Study the drawing (mm; zero at the part's minimum x, y, z) and answer. A direction names the side the tool comes from. Coordinates: 2 decimals unless noted, no trailing zeros. Write each loop counter-clockwise with the first axis right and the second up, starting at its lowest first coordinate (ties: lowest second). Pieces come first, ordered by that corner, then holes. Notation, with made-up numbers: (15, 16) -> (36, 16) arc R10 cw to (36, 24) -> close; hole circle Ø10 at (-21, -28). An arc over 180 degrees is marked (long way). Answer in a Markdown table with one row per item. Add a question column.
Item 1: For a pull along Y with two mould halves and no side action, classify the marked faces 1, 2 and 3 as +Y half, -Y half, draft (parallel to the pull), parting line (faces both ways), or undercut.
Item 2: Which of the six approach directions +Z, -Z, +X, -X, +Y, -Y give full straight-line access (tool end or side, diameter ignored) to the marked faces 4 and 5?
Item 3: Section B-B on z = 25 is taken. Write down the section's boundary in (x, y), then the cut area to 3 significant figures.
Item 4: Section D-D on x = 2 is taken. Write down the section's boundary in (y, z).
Item 5: Section C-C on y = 12.5 is taken. Write down the section's boundary in (x, z).
Item 6: Straight lines are drawn through the part: line 1 (Y direction, x = 8, z = 12.25); line 2 (Z direction, x = 5, y = 1); line 3 (Y direction, x = 9.75, z = 22) (1 decimal). For each, find the intervals that lie inside material, in ascending order. Write a range as from..to.
Item 7: Given pin 1 Ø3 at (x, z) = (7.5, 14) entering from -Y; pin 2 Ø1.5 at (x, y) = (7.5, 7) entering from -Z; pin 3 Ø1.5 at (x, z) = (6.5, 16) entering from -Y (1 decimal), each flat-ended and moving along its own axis, determine where each tip first touches the part or whether it passes through.
Item 8: Section A-A on x = 8 is taken. Write down the section's boundary in (y, z).
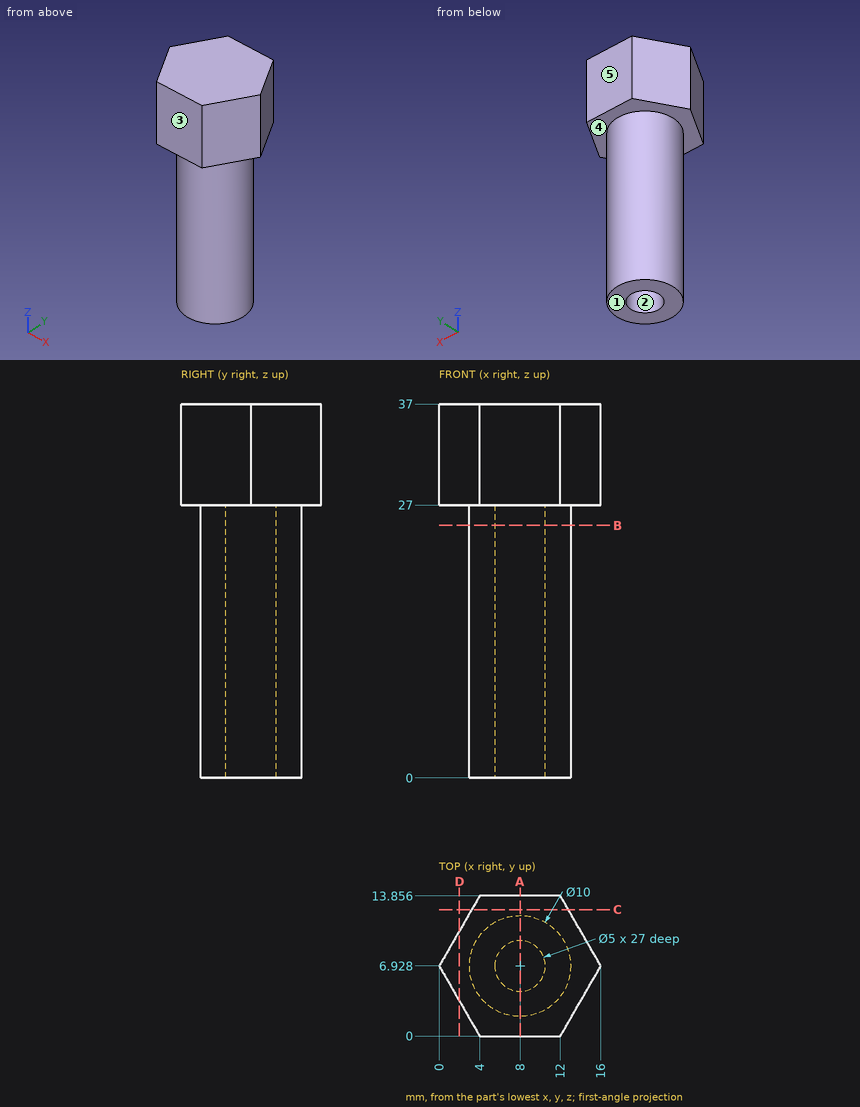
Results below:
| question | item | result |
|---|---|---|
| 1 | face 1 | draft |
| 1 | face 2 | undercut |
| 1 | face 3 | -Y half |
| 2 | face 4 | -Z |
| 2 | face 5 | +Z, -Z, +X, -X, +Y |
| 3 | outline | circle Ø10 at (8, 6.93); hole circle Ø5 at (8, 6.93) |
| 3 | area | 58.9 mm2 |
| 4 | outline | (3.46, 27) -> (10.39, 27) -> (10.39, 37) -> (3.46, 37) -> close |
| 5 | outline | (3.22, 27) -> (12.78, 27) -> (12.78, 37) -> (3.22, 37) -> close |
| 6 | line 1 | y = 1.93..4.43, 9.43..11.93 |
| 6 | line 2 | z = 27..37 |
| 6 | line 3 | y = 2.2..5.1, 8.7..11.6 |
| 7 | pin 1 | stops at y = 1.93 |
| 7 | pin 2 | stops at z = 27 |
| 7 | pin 3 | stops at y = 2 |
| 8 | outline | (0, 27) -> (1.93, 27) -> (1.93, 0) -> (4.43, 0) -> (4.43, 27) -> (9.43, 27) -> (9.43, 0) -> (11.93, 0) -> (11.93, 27) -> (13.86, 27) -> (13.86, 37) -> (0, 37) -> close |
